from build123d import *

# Parameters (mm, degrees)
CUT_EXTRUDE1_DEPTH = 38.749172176


with BuildPart() as part:
    # Sketch1 → Revolve1 (revolve)
    with BuildSketch(Plane.XY, mode=Mode.PRIVATE) as revolve1_sk:
        Polygon((0.75, 16), (-0.75, 16), (-3.059401077, 20), (-4, 20), (-4, 0), (4, 0), (21, 0), (21, 10), (16, 12), (4, 12), (4, 20), (3.059401077, 20), align=None)
    revolve(revolve1_sk.sketch.rotate(Axis((-19.792492436, 0, 0), (1, 0, 0)), 90), axis=Axis((-19.792492436, 0, 0), (1, 0, 0)))

    # Sketch2 → Cut-Extrude1 (cut, through all)
    with BuildSketch(Plane.ZY.offset(4)):
        with BuildLine():
            Line((-1.5, 8.337397166), (1.5, 8.337397166))
            Line((1.5, 8.337397166), (1.5, 6.837397166))
            ThreePointArc((1.5, 6.837397166), (0, -7), (-1.5, 6.837397166))
            Line((-1.5, 6.837397166), (-1.5, 8.337397166))
        make_face()
    extrude(amount=-CUT_EXTRUDE1_DEPTH, mode=Mode.SUBTRACT)


solid = part.part
Geometry: final body of the model. Coordinates: model frame, mm. A direction names the side the tool comes from. Coordinates: 2 decimals unless noted, no trailing zeros. Loops run counter-clockwise (first coordinate to the right, second up) from the corner with the lowest first, then second, coordinate; pieces in that order, holes last. Notation, with made-up numbers: (11.5, -27.75) - (45.5, -27.75) arc R18 ccw to (45.5, -2.75) - close; hole circle Ø1 at (61, 75.25). An arc over 180 degrees is marked (long way). Put each result on its own line as item: value. Start each with the question number.
Q1. Set-up query: faces 1 (the flat face through (8, 8, 1.5)), 2 (the flat face through (21, -7, -2)), 3 (the cylindrical face through (9.916, -3.604, 11.446)), 4 (the conical face through (-0.9, -4.9, 15.5)), 5 (the flat face through (-4, 0, 9)). Return all of +Z, -Z, +X, -X, +Y, -Y with unobstructed straight access to the full face (end or side cutting, diameter ignored); none if empty.
Q2. Pull-direction query (Y, two-part tool) for faces 6 (the cylindrical face through (8, -7, 0)), 7 (the flat face through (4, 9, -9)), 8 (the conical face through (0.862, -13.655, 8.706)); classes: released by +Y, released by -Y, zero draft, split by the parting line, or undercut.
Q3. Cut plane A-A, the plane z = 0. Return loops of the section in (x, y), and give its area (3 significant figures).
Q4. Cut plane D-D, the plane x = 11. Return loops of the section in (y, z), and give its area (3 significant figures).
Q5. Pin query (flat end, axial travel): pin 1 Ø1.5 at (x, y) = (0.5, -2.5) entering from +Z; pin 2 Ø12 at (x, z) = (5, -4.5) entering from -Y; pin 3 Ø5 at (x, z) = (11, -3) entering from -Y; pin 4 Ø4 at (x, z) = (8.5, 15.5) entering from +Y. Return the tip coordinate at first contact, or that it passes through.
Q6. Cut plane C-C, the plane x = 16.5. Return loops of the section in (y, z).
Q7. Line query: line 1 (Y direction, x = 8.75, z = 0); line 2 (X direction, y = -8, z = 10.5); line 3 (Z direction, x = 4.25, y = 3.5). Output: solid intervals per line, ascending.
Q8. Cut plane B-B, the plane y = 0. Return loops of the section in (x, z), and give its area (3 significant figures).
Filled sheet:
1. face 1: +X, -X
1. face 2: +Z, -Z, +X, +Y, -Y
1. face 3: +X
1. face 4: none
1. face 5: +Z, -Z, -X, +Y, -Y
2. face 6: undercut
2. face 7: zero draft
2. face 8: split by the parting line
3. outline: (-4, -20) - (-3.06, -20) - (-0.75, -16) - (0.75, -16) - (3.06, -20) - (4, -20) - (4, -12) - (16, -12) - (21, -10) - (21, -7) - (-4, -7) - close; (-4, 8.34) - (21, 8.34) - (21, 10) - (16, 12) - (4, 12) - (4, 20) - (3.06, 20) - (0.75, 16) - (-0.75, 16) - (-3.06, 20) - (-4, 20) - close
3. area: 304 mm²
4. outline: circle Ø24 at (0, 0); hole (6.84, -1.5) - (8.34, -1.5) - (8.34, 1.5) - (6.84, 1.5) arc R7 ccw (long way) to start
4. area: 294 mm²
5. pin 1: z = 16.68
5. pin 2: y = -20
5. pin 3: y = -11.99
5. pin 4: through
6. outline: circle Ø23.6 at (0, 0); hole (6.84, -1.5) - (8.34, -1.5) - (8.34, 1.5) - (6.84, 1.5) arc R7 ccw (long way) to start
7. line 1: -12 to -7, 8.34 to 12
7. line 2: -4 to 4
7. line 3: -11.48 to -6.06, 6.06 to 11.48
8. outline: (-4, -20) - (-3.06, -20) - (-0.75, -16) - (0.75, -16) - (3.06, -20) - (4, -20) - (4, -12) - (16, -12) - (21, -10) - (21, -7) - (-4, -7) - close; (-4, 7) - (21, 7) - (21, 10) - (16, 12) - (4, 12) - (4, 20) - (3.06, 20) - (0.75, 16) - (-0.75, 16) - (-3.06, 20) - (-4, 20) - close
8. area: 338 mm²
